Read the model definition and answer for the solid it produces. Units are mm, in the model's axes. A direction names the side the tool comes from. Give positions to 0.01 mm unless a question says otherwise; leave off trailing zeros. Write each loop counter-clockwise with the first axis right and the second up, starting at its lowest first coordinate (ties: lowest second). Pieces come first, ordered by that corner, then holes. Notation, with made-up numbers: M -20.5,-34 L -11.5,-34 A14 cw -11.5,-29 Z; hole C 53.25,17 d11. An arc over 180 degrees is marked long. Use a Markdown table: item, result. Add a question column.
Item 1: A cutting plane is placed at A-A on y = 319. Determine the outline of the cut face in (x, z), then the cut area to 3 significant figures.
Item 2: Consider probe 1 along Z at (x, y) = (5.5, 641); probe 2 along X at (y, z) = (410, 9.45). Determine where each line is inside the solid, lowest interval first. Write a range as [from, to].
Item 3: A cutting plane is placed at B-B on z = 5.75. Determine the outline of the cut face in (x, y).
Item 4: For faces 1 (the flat face through (0, 456, 10)), 2 (the flat face through (9, 456, 0)), determine the directions among +Z, -Z, +X, -X, +Y, -Y from which every point of the face is accessible in a straight line to the end or side of a thin tool.
Item 5: The mould has two halves that part along X. Classify faces 3 (the flat face through (-0.8, 740, 9.6)), 4 (the flat face through (10, 456, 0)), 5 (the flat face through (-9, 456, 0)): pulls with the +X half, pulls with the -X half, needs draft (parallel to the pull), parting line crosses it, or undercut.
from build123d import *

# Parameters (mm, degrees)
SKETCH_1_W          = 20
SKETCH_1_H          = 20
SKETCH_1_W_2        = 18
SKETCH_1_H_2        = 18
EXTRUDE_1_DEPTH     = 740
SKETCH_3_R          = 1.65
CUT_EXTRUDE_1_DEPTH = 32
SKETCH_4_R          = 1.65
CUT_EXTRUDE_2_DEPTH = 741.337760755
SKETCH_5_R          = 14.566227152
CUT_EXTRUDE_3_DEPTH = 180
SKETCH_6_R          = 1.65
CUT_EXTRUDE_4_DEPTH = 30
SKETCH_7_R          = 1.65
CUT_EXTRUDE_5_DEPTH = 741.337760755


with BuildPart() as part:
    # 草图1 → 凸台-拉伸1 (new body)
    with BuildSketch(Plane(origin=(0, 0, 0), x_dir=(1, 0, 0), z_dir=(0, 1, 0))):
        Rectangle(SKETCH_1_W, SKETCH_1_H)
        Rectangle(SKETCH_1_W_2, SKETCH_1_H_2, mode=Mode.SUBTRACT)
    extrude(amount=EXTRUDE_1_DEPTH)

    # 草图3 → 切除-拉伸1 (cut)
    with BuildSketch(Plane.XY.offset(10)):
        with Locations((0, 720)):
            Circle(SKETCH_3_R)
        with Locations((0, 700)):
            Circle(SKETCH_3_R)
        with Locations((0, 680)):
            Circle(SKETCH_3_R)
        with Locations((0, 660)):
            Circle(SKETCH_3_R)
        with Locations((0, 590)):
            Circle(SKETCH_3_R)
        with Locations((0, 570)):
            Circle(SKETCH_3_R)
        with Locations((0, 550)):
            Circle(SKETCH_3_R)
        with Locations((0, 450)):
            Circle(SKETCH_3_R)
        with Locations((0, 430)):
            Circle(SKETCH_3_R)
        with Locations((0, 410)):
            Circle(SKETCH_3_R)
    extrude(amount=-CUT_EXTRUDE_1_DEPTH, mode=Mode.SUBTRACT)

    # 草图4 → 切除-拉伸2 (cut, through all)
    with BuildSketch(Plane(origin=(10, 0, 0), x_dir=(0, 0, -1), z_dir=(1, 0, 0))):
        with Locations((0, 250)):
            Circle(SKETCH_4_R)
        with Locations((0, 270)):
            Circle(SKETCH_4_R)
        with Locations((0, 290)):
            Circle(SKETCH_4_R)
        with Locations((0, 310)):
            Circle(SKETCH_4_R)
    extrude(amount=-CUT_EXTRUDE_2_DEPTH, mode=Mode.SUBTRACT)

    # 草图5 → 切除-拉伸3 (cut)
    with BuildSketch(Plane.XZ):
        Circle(SKETCH_5_R)
    extrude(amount=-CUT_EXTRUDE_3_DEPTH, mode=Mode.SUBTRACT)

    # 草图6 → 切除-拉伸4 (cut)
    with BuildSketch(Plane(origin=(10, 0, 0), x_dir=(0, 0, -1), z_dir=(1, 0, 0))):
        with Locations((0, 190)):
            Circle(SKETCH_6_R)
        with Locations((0, 200)):
            Circle(SKETCH_6_R)
        with Locations((0, 210)):
            Circle(SKETCH_6_R)
    extrude(amount=-CUT_EXTRUDE_4_DEPTH, mode=Mode.SUBTRACT)

    # 草图7 → 切除-拉伸5 (cut, through all)
    with BuildSketch(Plane(origin=(0, 0, -10), x_dir=(-1, 0, 0), z_dir=(0, 0, -1))):
        with Locations((0, 195)):
            Circle(SKETCH_7_R)
        with Locations((0, 205)):
            Circle(SKETCH_7_R)
        with Locations((0, 215)):
            Circle(SKETCH_7_R)
    extrude(amount=-CUT_EXTRUDE_5_DEPTH, mode=Mode.SUBTRACT)


solid = part.part
Filled in:
| question | item | result |
|---|---|---|
| 1 | outline | M -10,-10 L 10,-10 L 10,10 L -10,10 Z; hole M -9,-9 L 9,-9 L 9,9 L -9,9 Z |
| 1 | area | 76.0 mm² |
| 2 | probe 1 | [-10, -9], [9, 10] |
| 2 | probe 2 | [-10, -1.65], [1.65, 10] |
| 3 | outline | M -10,180 L -9,180 L -9,740 L -10,740 Z; M 9,180 L 10,180 L 10,740 L 9,740 Z |
| 4 | face 1 | +Z, +X, -X, +Y, -Y |
| 4 | face 2 | +Y, -Y |
| 5 | face 3 | needs draft |
| 5 | face 4 | pulls with the +X half |
| 5 | face 5 | undercut |
